Design review of the part built by this model. Coordinates are the model's own, in mm. Face numbers are marked on the shaded views. A direction names the side the tool comes from. Round coordinates to 2 decimals unless told otherwise and drop trailing zeros. Loops run counter-clockwise (first coordinate to the right, second up) from the corner with the lowest first, then second, coordinate; pieces in that order, holes last. Notation, with made-up numbers: (38.25, 21) - (92.25, 21) arc R16 ccw to (92.25, 28) - close; hole circle Ø9 at (28.25, 85.5). An arc over 180 degrees is marked (long way). Return JSON: item names as keys, results as strings. Group by question number.
(1) We need section A-A, the plane x = 0. Give the number of separate pieces and of enclosed holes in the cut face, and give its area (3 significant figures).
(2) We need section C-C, the plane y = 20.5. Write out the cut boundary in (x, z).
(3) Clearance check with flat-ended pins moving along their axes: pin 1 (2.5 mm diameter, centred on x = -17.75, y = -10.25, fed in from +Z); pin 2 (6.5 mm diameter, centred on y = 13.5, z = 10.5, fed in from +X); pin 3 (8 mm diameter, centred on x = -9.5, y = 8, fed in from +Z); pin 4 (1 mm diameter, centred on y = 0, z = 14, fed in from -X). State where each tip first meets the part, or that it passes through.
(4) For the marked faces 1 and 2, list the 3-axis set-ups (+Z, -Z, +X, -X, +Y, -Y) from which the entire face can be reached by the end or side of a thin tool; tool diameter is ignored.
(5) The part is to be moulded in two halves that separate along Y. For the marked faces 3, 4 and 5, say which applies: pulls with the +Y half, pulls with the -Y half, needs draft (parallel to the pull), parting line crosses it, or undercut.
(6) Wall thickness on L1, parallel to Y at x = 10.5, z = 9.75; L2, parallel to Y at x = 3, z = 6; L3, parallel to Z at x = -18.5, y = 16.5: over which ranges is each line inside the solid? List them lowest first. Write a range as [from, to].
from build123d import *

# Parameters (mm, degrees)
F3_DEPTH      = 25
F3_DEPTH_BACK = 9
F4_R          = 0.9
F5_DEPTH      = 22.001


with BuildPart() as f1:
    # F0 (on Front) → F1 (revolve)
    with BuildSketch(Plane.XZ):
        Polygon((4.5, 0), (27, 0), (27, 4.6), (26, 4.6), (26, 3), (23, 3), (23, 12), (18, 12), (10, 12), (10, 22), (4.5, 22), align=None)
        Polygon((18, 12), (10, 22), (10, 12), align=None)
    revolve(axis=Axis((0, 0, 11.323432), (0, 0, 1)))

    # F2 (on face) → F3 (cut, two sides)
    with BuildSketch(Plane.XY.offset(12)) as f3_sk:
        with BuildLine():
            ThreePointArc((-7.135255, 7.006293), (-5, 8.660254), (-2.5, 9.682458))
            Line((-2.5, 9.682458), (-2.5, 17.825543))
            ThreePointArc((-2.5, 17.825543), (-9, 15.588457), (-14.187373, 11.077835))
            Line((-14.187373, 11.077835), (-7.135255, 7.006293))
        make_face()
        with BuildLine():
            ThreePointArc((-9.635255, -2.676166), (-10, 0), (-9.635255, 2.676166))
            Line((-9.635255, 2.676166), (-16.687373, 6.747708))
            ThreePointArc((-16.687373, 6.747708), (-18, 0), (-16.687373, -6.747708))
            Line((-16.687373, -6.747708), (-9.635255, -2.676166))
        make_face()
        with BuildLine():
            Line((-2.5, -17.825543), (-2.5, -9.682458))
            ThreePointArc((-2.5, -9.682458), (-5, -8.660254), (-7.135255, -7.006293))
            Line((-7.135255, -7.006293), (-14.187373, -11.077835))
            ThreePointArc((-14.187373, -11.077835), (-9, -15.588457), (-2.5, -17.825543))
        make_face()
        with BuildLine():
            Line((14.187373, -11.077835), (7.135255, -7.006293))
            ThreePointArc((7.135255, -7.006293), (5, -8.660254), (2.5, -9.682458))
            Line((2.5, -9.682458), (2.5, -17.825543))
            ThreePointArc((2.5, -17.825543), (9, -15.588457), (14.187373, -11.077835))
        make_face()
        with BuildLine():
            ThreePointArc((9.635255, 2.676166), (9.908394, 1.350454), (10, 0))
            ThreePointArc((10, 0), (9.908394, -1.350454), (9.635255, -2.676166))
            Line((9.635255, -2.676166), (16.687373, -6.747708))
            ThreePointArc((16.687373, -6.747708), (17.668796, -3.437097), (18, 0))
            ThreePointArc((18, 0), (17.668796, 3.437097), (16.687373, 6.747708))
            Line((16.687373, 6.747708), (9.635255, 2.676166))
        make_face()
        with BuildLine():
            ThreePointArc((2.5, 9.682458), (5, 8.660254), (7.135255, 7.006293))
            Line((7.135255, 7.006293), (14.187373, 11.077835))
            ThreePointArc((14.187373, 11.077835), (9, 15.588457), (2.5, 17.825543))
            Line((2.5, 17.825543), (2.5, 9.682458))
        make_face()
    extrude(amount=F3_DEPTH, mode=Mode.SUBTRACT)
    extrude(f3_sk.sketch, amount=-F3_DEPTH_BACK, mode=Mode.SUBTRACT)

    # F4 (on face) → F5 (cut, through all)
    with BuildSketch(Plane.XY.offset(22)):
        with Locations((0, 7)):
            Circle(F4_R)
        with Locations((0, 20.5)):
            Circle(F4_R)
        with Locations((-6.062178, 3.5)):
            Circle(F4_R)
        with Locations((-17.753521, 10.25)):
            Circle(F4_R)
        with Locations((-6.062178, -3.5)):
            Circle(F4_R)
        with Locations((-17.753521, -10.25)):
            Circle(F4_R)
        with Locations((0, -7)):
            Circle(F4_R)
        with Locations((0, -20.5)):
            Circle(F4_R)
        with Locations((6.062178, -3.5)):
            Circle(F4_R)
        with Locations((17.753521, -10.25)):
            Circle(F4_R)
        with Locations((6.062178, 3.5)):
            Circle(F4_R)
        with Locations((17.753521, 10.25)):
            Circle(F4_R)
    extrude(amount=-F5_DEPTH, mode=Mode.SUBTRACT)


solid = f1.part
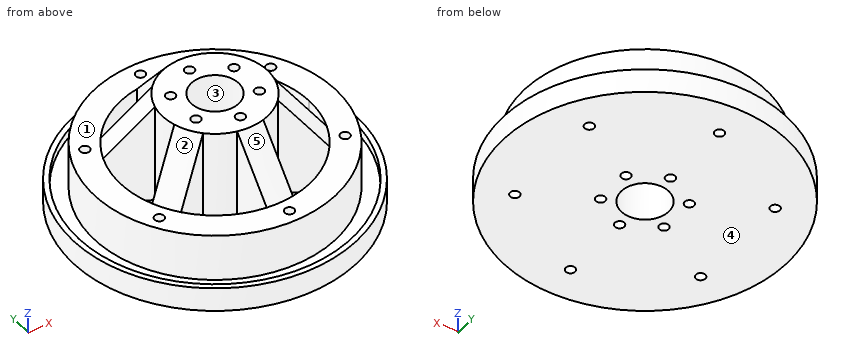
Solutions:
{
 "1": {"separate pieces": "6", "enclosed holes": "0", "area": "539 mm^2"},
 "2": {"outline": "(-17.57, 0) - (-0.9, 0) - (-0.9, 12) - (-10.43, 12) - (-10.43, 3) - (-15.99, 3) - (-15.99, 4.6) - (-17.57, 4.6) - close; (0.9, 0) - (17.57, 0) - (17.57, 4.6) - (15.99, 4.6) - (15.99, 3) - (10.43, 3) - (10.43, 12) - (0.9, 12) - close"},
 "3": {"pin 1": "z = 12", "pin 2": "x = 20.59", "pin 3": "z = 22", "pin 4": "x = -10"},
 "4": {"face 1": "+Z", "face 2": "+Z, -X, -Y"},
 "5": {"face 3": "undercut", "face 4": "needs draft", "face 5": "pulls with the -Y half"},
 "6": {"L1": "[-20.46, -14.62], [-8.95, -3.18], [3.18, 8.95], [14.62, 20.46]", "L2": "[-22.8, -17.75], [-9.54, -3.35], [3.35, 9.54], [17.75, 22.8]", "L3": "[0, 3]"}
}
